```python
from build123d import *

# Parameters (mm, degrees)
CYLINDER_R          = 1.75
CYLINDER_DEPTH      = 20
CYLINDER_ROLL_ANGLE = -90
PAD006_DEPTH        = 10
FILLET_R            = 4.9
CHAMFER_SIZE        = 1


with BuildPart() as cylinder:
    # Cylinder → Cylinder (new body)
    with BuildSketch(Plane.XY):
        Circle(CYLINDER_R)
    extrude(amount=CYLINDER_DEPTH)


with BuildPart() as cylinder_1:
    # Cylinder roll: moved
    add(cylinder.part.rotate(Axis((0, 0, 0), (1, 0, 0)), CYLINDER_ROLL_ANGLE))


with BuildPart() as cylinder_2:
    # Cylinder placement: moved
    add(cylinder_1.part.moved(Location((12, -10, 5))))


with BuildPart() as chamfer_body:
    # Sketch005 → Pad006 (new body)
    with BuildSketch(Plane.XY):
        with BuildLine():
            ThreePointArc((3, 4), (-5, 0), (3, -4))
            Line((17, -4), (3, -4))
            Line((17, -7), (17, -4))
            Line((0, -7), (17, -7))
            ThreePointArc((0, 7), (-7, 0), (0, -7))
            Line((0, 7), (17, 7))
            Line((17, 4), (17, 7))
            Line((3, 4), (17, 4))
        make_face()
    extrude(amount=PAD006_DEPTH)

    # Cut004: cut Cylinder
    add(cylinder_2.part, mode=Mode.SUBTRACT)

    # Fillet
    fillet_edges = [chamfer_body.edges().sort_by_distance(p)[0] for p in [
        (17, -5.5, 0),
        (17, 5.5, 0),
        (17, -5.5, 10),
        (17, 5.5, 10),
    ]]
    fillet(fillet_edges, radius=FILLET_R)

    # Chamfer
    chamfer_edges = [chamfer_body.edges().sort_by_distance(p)[0] for p in [
        (6.05, -7, 10),
    ]]
    chamfer(chamfer_edges, length=CHAMFER_SIZE)


solid = chamfer_body.part
```
Work out the finished part from the listing and answer in its coordinate system (mm). A direction names the side the tool comes from. Coordinates: 2 decimals unless noted, no trailing zeros. Loops run counter-clockwise (first coordinate to the right, second up) from the corner with the lowest first, then second, coordinate; pieces in that order, holes last. Notation, with made-up numbers: M 81.25,14.25 L 121.25,14.25 A17 ccw 121.25,22.25 Z; hole C -12,57.5 d1. An arc over 180 degrees is marked long. Use CSV: the item, a comma, the result in double quotes. Start each with the question number.
(1) Consider line 1 (Y direction, x = 11.75, z = 7); line 2 (Z direction, x = 12, y = 5.35); line 3 (Y direction, x = 0, z = 5.5). Determine where each line is inside the solid, lowest interval first.
(2) For faces 5 (the face through (10, -4, 5)), 6 (the face through (15.08, 6.73, 8.02)), determine the directions among +Z, -Z, +X, -X, +Y, -Y from which every point of the face is accessible in a straight line to the end or side of a thin tool.
(3) Given pin 1 Ø5 at (y, z) = (-1, 5) entering from +X; pin 2 Ø6 at (y, z) = (0, 6.5) entering from +X; pin 3 Ø6 at (y, z) = (5, 9) entering from +X, each flat-ended and moving along its own axis, determine where each tip first touches the part or whether it passes through.
(4) Find section C-C, the plane z = 4.25. State how many separate pieces and enclosed holes the cut face has, then the cut area to 3 significant figures.
(5) Find section B-B, the plane y = 0. Give the vertices of the cut face in (x, z), then the cut area to 3 significant figures.
(6) Find section A-A, the plane x = 8.5. Give the vertices of the cut face in (y, z).
(7) For a pull along Z with two mould halves and no side action, classify faces 1 (the face through (13.669, 5.479, 4.474)), 2 (the face through (10, 4, 5)), 3 (the face through (15.53, -4.99, 1.4)), 4 (the face through (15.53, -4.99, 8.6)) as +Z half, -Z half, draft (parallel to the pull), parting line (faces both ways), or undercut.
Recorded:
1,line 1,"y = -7 to -4, 4 to 7"
1,line 2,"z = 0 to 3.25, 6.75 to 10"
1,line 3,"y = -7 to -5, 5 to 7"
2,face 5,"+Z, -Z, +X"
2,face 6,"+Z, +X, +Y"
3,pin 1,"stops at x = -3.57"
3,pin 2,"stops at x = -4"
3,pin 3,"stops at x = 16.92"
4,separate pieces,"3"
4,enclosed holes,"0"
4,area,"115 mm^2"
5,outline,"M -7,1 L -6,0 L -5,0 L -5,10 L -6,10 L -7,9 Z"
5,area,"19.0 mm^2"
6,outline,"M -7,1 L -6,0 L -4,0 L -4,10 L -6,10 L -7,9 Z; M 4,0 L 6,0 L 7,1 L 7,9 L 6,10 L 4,10 Z"
7,face 1,"undercut"
7,face 2,"draft"
7,face 3,"-Z half"
7,face 4,"+Z half"
